```python
from build123d import *

# Parameters (mm, degrees)
F0_W     = 360
F0_H     = 150
F1_DEPTH = 20
F3_DEPTH = 20
F4_W     = 340
F4_H     = 4
F5_DEPTH = 3


with BuildPart() as f1:
    # F0 (on Front) → F1 (new body)
    with BuildSketch(Plane.XZ):
        with Locations((-7.764109, -54.714244)):
            Rectangle(F0_W, F0_H)
    extrude(amount=F1_DEPTH)

    # F2 (on face) → F3 (cut)
    with BuildSketch(Plane.XZ.offset(20)):
        Polygon((172.235891, -27.214244), (152.235891, -22.214244), (152.235891, -47.214244), (172.235891, -42.214244), align=None)
        Polygon((172.235891, -67.214244), (152.235891, -62.214244), (152.235891, -87.214244), (172.235891, -82.214244), align=None)
        Polygon((152.235891, -102.212298), (152.235891, -127.216189), (172.235891, -122.214244), (172.235891, -107.214244), align=None)
        Polygon((172.235891, 12.785756), (152.235891, 17.787702), (152.235891, -7.216189), (172.235891, -2.214244), align=None)
        Polygon((172.235891, 20.285756), (152.235891, 20.285756), (152.235891, 17.787702), (172.235891, 12.785756), align=None)
        Polygon((152.235891, -127.216189), (152.235891, -129.714244), (172.235891, -129.714244), (172.235891, -122.214244), align=None)
    extrude(amount=-F3_DEPTH, mode=Mode.SUBTRACT)

    # F4 (on face) → F5 (cut)
    with BuildSketch(Plane.XZ.offset(20)):
        with Locations((-17.764109, -121.714244)):
            Rectangle(F4_W, F4_H)
    extrude(amount=-F5_DEPTH, mode=Mode.SUBTRACT)


solid = f1.part
```
For this review, take the finished solid that the model builds, in its own axes (mm). A direction names the side the tool comes from. Coordinates: 2 decimals unless noted, no trailing zeros. Write each loop counter-clockwise with the first axis right and the second up, starting at its lowest first coordinate (ties: lowest second). Pieces come first, ordered by that corner, then holes.
(1) The part is to be moulded in two halves that separate along X. For faces 1 (the face through (-20, -10, 20.286)), 2 (the face through (172.236, -10, -15)), 3 (the face through (152.236, -10, -116)), say which applies: +X half, -X half, draft (parallel to the pull), parting line (faces both ways), or undercut.
(2) Tool access review of faces 4 (the face through (-187.764, -10, -56)), 5 (the face through (172.236, -10, -55)), 6 (the face through (152.236, -10, 7)), 7 (the face through (162.38, -10.14, -104.75)), 8 (the face through (162.38, -10.14, -64.75)): name each direction out of +Z, -Z, +X, -X, +Y, -Y from which nothing blocks a thin tool from reaching the whole face with its end or side.
(3) For pin 1 Ø10 at (y, z) = (-15, -76) entering from +X, flat-tipped, find the tip position at first contact; note if it passes through.
(4) Add section B-B on z = -72. Give the boundary of the cut face in (x, y).
(5) Add section A-A on y = -8. Give the boundary of the cut face in (x, z).
(6) Wall thickness on probe 1 along X at (y, z) = (-1, -31.5): over which ranges is the line inside the solid? List them lowest first.
Answer sheet:
1. face 1: draft
1. face 2: +X half
1. face 3: undercut
2. face 4: +Z, -Z, -X, +Y, -Y
2. face 5: +Z, -Z, +X, +Y, -Y
2. face 6: +Z, +Y, -Y
2. face 7: -Z, +Y, -Y
2. face 8: +Y, -Y
3. pin 1: stops at x = 152.24
4. outline: (-187.76, -20) - (152.24, -20) - (152.24, 0) - (-187.76, 0) - close
5. outline: (-187.76, -129.71) - (152.24, -129.71) - (152.24, -102.21) - (172.24, -107.21) - (172.24, -82.21) - (152.24, -87.21) - (152.24, -62.21) - (172.24, -67.21) - (172.24, -42.21) - (152.24, -47.21) - (152.24, -22.21) - (172.24, -27.21) - (172.24, -2.21) - (152.24, -7.22) - (152.24, 20.29) - (-187.76, 20.29) - close
6. probe 1: x = -187.76 to 152.24
